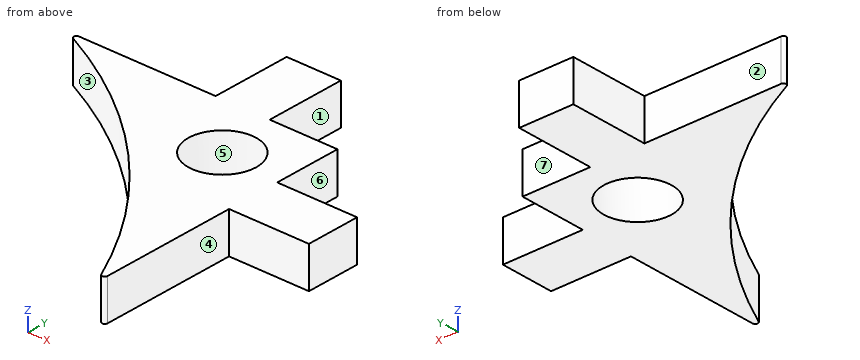
Autodesk Inventor part; units mm, degrees
ref_plane "YZ Plane" through (0, 0, 0) normal (1, 0, 0) x (0, 1, 0)
ref_plane "XZ Plane" through (0, 0, 0) normal (0, 1, 0) x (-1, 0, 0)
ref_plane "XY Plane" through (0, 0, 0) normal (0, 0, 1) x (1, 0, 0)
sketch "Sketch1" plane through (0, 0, 0) normal (0, 0, 1) x (1, 0, 0)
  arc A0 (0, -20) -> (-20, 0) centre (-36.4575, -36.4575) ccw
  circle A1 centre (-4.5, -4.5) radius 2.5
  line L0 (-20, 0) -> (-9, 0)
  line L1 (-9, 0) -> (-9, 5.9)
  line L2 (-9, 5.9) -> (-5, 5.9)
  line L3 (-5, 5.9) -> (-5, 0)
  line L4 (-5, 0) -> (0, 0)
  line L5 (0, 0) -> (0, -5)
  line L6 (0, -5) -> (5.9, -5)
  line L7 (5.9, -5) -> (5.9, -9)
  line L8 (5.9, -9) -> (0, -9)
  line L9 (0, -9) -> (0, -20)
  dimension "d0" = 20
  dimension "d1" = 20
  dimension "d2" = 40
  dimension "d5" = 5
  dimension "d9" = 4
  dimension "d10" = 5.9
  dimension "d12" = 4.5
  dimension "d13" = 5.9
  dimension "d14" = 4
  dimension "d17" = 5
  dimension "d18" = 4.5
  dimension "d19" = 5
extrude "Extrusion1" add sketch "Sketch1" along normal blind 3
fillet "Fillet1" radius 0.2 2 edges at (0, -20, 1.5) (-20, 0, 1.5)
properties part number "Gripper V 8.0 servo support bracket"
For this review, take the finished solid that the model builds, in its own axes (mm). Face numbers are marked on the shaded views. A direction names the side the tool comes from. Coordinates: 2 decimals unless noted, no trailing zeros. Write each loop counter-clockwise with the first axis right and the second up, starting at its lowest first coordinate (ties: lowest second). Pieces come first, ordered by that corner, then holes. Notation, with made-up numbers: (24, 70) -> (59, 70) arc R34 ccw to (59, 105) -> close; hole circle Ø6 at (27, 40). An arc over 180 degrees is marked (long way). Write each question's results on one line, items separated by ' | '. Start each with the question number.
1) Consider section A-A (z = 2.45). Write out the cut boundary in (x, y), plus the area to 3 significant figures.
2) The part is to be moulded in two halves that separate along X. For the marked faces 5, 6 and 7, say which applies: +X half, -X half, draft (parallel to the pull), parting line (faces both ways), or undercut.
3) Consider section D-D (x = -9.75). Write out the cut boundary in (y, z), plus the area to 3 significant figures.
4) Wall thickness on L1, parallel to Y at x = 4, z = 0.4; L2, parallel to Y at x = -4.5, z = 2; L3, parallel to X at y = -2.5, z = 1.2: over which ranges is each line inside the solid? List them lowest first. Write a range as [from, to].
5) For the marked faces 1, 2, 3 and 4, list the 3-axis set-ups (+Z, -Z, +X, -X, +Y, -Y) from which the entire face can be reached by the end or side of a thin tool; tool diameter is ignored.
6) Consider section C-C (y = -3.25). Write out the cut boundary in (x, z), plus the area to 3 significant figures.
7) Insertion check: pin 1 (0.9 mm diameter, centred on x = -13.5, z = 2, fed in from +Y); pin 2 (1.5 mm diameter, centred on y = 3, z = 2, fed in from -X); pin 3 (0.9 mm diameter, centred on y = -1.5, z = 2, fed in from +X); pin 4 (4.5 mm diameter, centred on x = -4.5, y = -4.5, fed in from +Z). Each pin has a flat end and moves straight along its axis. Give the tip position at first contact, or say it passes through.
8) Consider section B-B (x = -4.5). Write out the cut boundary in (y, z), plus the area to 3 significant figures.
Geometry says:
1) outline: (-19.18, -0.38) arc R40 cw to (-0.38, -19.18) arc R0.2 ccw to (0, -19.1) -> (0, -9) -> (5.9, -9) -> (5.9, -5) -> (0, -5) -> (0, 0) -> (-5, 0) -> (-5, 5.9) -> (-9, 5.9) -> (-9, 0) -> (-19.1, 0) arc R0.2 ccw to start; hole circle Ø5 at (-4.5, -4.5) | area: 178 mm^2
2) face 5: undercut | face 6: +X half | face 7: draft
3) outline: (-6.68, 0) -> (0, 0) -> (0, 3) -> (-6.68, 3) -> close | area: 20.0 mm^2
4) L1: [-9, -5] | L2: [-12.4, -7], [-2, 0] | L3: [-15.32, -6], [-3, 0]
5) face 1: +Z, -Z, +X, +Y | face 2: +Z, -Z, -X, +Y | face 3: +Z, -Z, -X, -Y | face 4: +Z, -Z, +X, -Y
6) outline: (-14.16, 0) -> (-6.67, 0) -> (-6.67, 3) -> (-14.16, 3) -> close; (-2.33, 0) -> (0, 0) -> (0, 3) -> (-2.33, 3) -> close | area: 29.5 mm^2
7) pin 1: y = 0 | pin 2: x = -9 | pin 3: x = 0 | pin 4: through
8) outline: (-12.4, 0) -> (-7, 0) -> (-7, 3) -> (-12.4, 3) -> close; (-2, 0) -> (0, 0) -> (0, 3) -> (-2, 3) -> close | area: 22.2 mm^2
